```python
from build123d import *

# Parameters (mm, degrees)
EXTRUDE_1_DEPTH     = 20
EXTRUDE_2_DEPTH     = 8
CUT_EXTRUDE_1_DEPTH = 35.756294394
SKETCH_4_R          = 1.6
CUT_EXTRUDE_2_DEPTH = 37.307712679


with BuildPart() as part:
    # ｽｹｯﾁ1 → ﾎﾞｽ - 押し出し1 (new body)
    with BuildSketch(Plane(origin=(0, 0, 0), x_dir=(1, 0, 0), z_dir=(0, 1, 0))):
        with BuildLine():
            Line((-4.5, -8.93028555), (-4.5, -18))
            Line((-4.5, -18), (4.5, -18))
            Line((4.5, -18), (4.5, -8.93028555))
            ThreePointArc((4.5, -8.93028555), (0, 10), (-4.5, -8.93028555))
        make_face()
    extrude(amount=EXTRUDE_1_DEPTH)

    # ｽｹｯﾁ2 → ﾎﾞｽ - 押し出し2 (add)
    with BuildSketch(Plane(origin=(0, 20, 0), x_dir=(1, 0, 0), z_dir=(0, 1, 0))):
        Polygon((0, 5.773502692), (-5, 2.886751346), (-5, -2.886751346), (0, -5.773502692), (5, -2.886751346), (5, 2.886751346), align=None)
    extrude(amount=EXTRUDE_2_DEPTH)

    # ｽｹｯﾁ3 → ｶｯﾄ - 押し出し1 (cut, through all)
    with BuildSketch(Plane(origin=(0, 28, 0), x_dir=(1, 0, 0), z_dir=(0, 1, 0))):
        with BuildLine():
            Line((-3.638778503, -18), (-0.312080176, -1.543771668))
            ThreePointArc((-0.312080176, -1.543771668), (0, 1.575), (0.312080176, -1.543771668))
            Line((0.312080176, -1.543771668), (3.638778503, -18))
            ThreePointArc((3.638778503, -18), (0, -18.364114708), (-3.638778503, -18))
        make_face()
    extrude(amount=-CUT_EXTRUDE_1_DEPTH, mode=Mode.SUBTRACT)

    # ｽｹｯﾁ4 → ｶｯﾄ - 押し出し2 (cut, through all)
    with BuildSketch(Plane.ZY.offset(4.5)):
        with Locations((13.465142775, 15)):
            Circle(SKETCH_4_R)
        with Locations((13.465142775, 5)):
            Circle(SKETCH_4_R)
    extrude(amount=-CUT_EXTRUDE_2_DEPTH, mode=Mode.SUBTRACT)


solid = part.part
```
Input: part model. Units: mm. Frame: model coordinates. A direction names the side the tool comes from. Give positions to 0.01 mm unless a question says otherwise; leave off trailing zeros. Order: outer loops, then holes, each group sorted by start corner. A loop starts at its lowest first (then second) coordinate and runs counter-clockwise, first axis right, second up. Notation, with made-up numbers: (45.5, 52) - (67.5, 52) arc R12 ccw to (67.5, 58) - close; hole circle Ø1 at (20, 22). An arc over 180 degrees is marked (long way). Use a Markdown table: item, result.
(1) Section query D-D (z = 10.5). Output: boundary loops of the cut face in (x, y), then the cut area to 3 significant figures.
Computed values:
| item | result |
|---|---|
| outline | (-4.5, 0) - (-2.12, 0) - (-2.12, 20) - (-4.5, 20) - close; (2.12, 0) - (4.5, 0) - (4.5, 20) - (2.12, 20) - close |
| area | 95.1 mm2 |
(2) Section query A-A (z = 0). Output: boundary loops of the cut face in (x, y) (3 decimals), then the cut area to 3 significant figures.
Computed values:
| item | result |
|---|---|
| outline | (-10, 0) - (-1.575, 0) - (-1.575, 28) - (-5, 28) - (-5, 20) - (-10, 20) - close; (1.575, 0) - (10, 0) - (10, 20) - (5, 20) - (5, 28) - (1.575, 28) - close |
| area | 392 mm2 |
(3) Pin query (flat end, axial travel): pin 1 (4.5 mm diameter, centred on y = 14, z = 12, fed in from +X); pin 2 (12 mm diameter, centred on x = 0.5, z = -0.5, fed in from -Y); pin 3 (5 mm diameter, centred on y = 15, z = 13.47, fed in from -X); pin 4 (4.5 mm diameter, centred on y = 25, z = 1.5, fed in from -X). Return the tip coordinate at first contact, or that it passes through.
Computed values:
| item | result |
|---|---|
| pin 1 | stops at x = 4.5 |
| pin 2 | stops at y = 0 |
| pin 3 | stops at x = -4.5 |
| pin 4 | stops at x = -5 |
(4) Draft query along Y for faces 5 (the flat face through (4, 20, 4)), 6 (the cylindrical face through (3.656, 15.07, 11.867)), 7 (the cylindrical face through (-3.686, 15.07, 11.867)), 8 (the flat face through (4.5, 10, 14)). Return one class per face: released by +Y, released by -Y, zero draft, split by the parting line, or undercut.
Computed values:
| item | result |
|---|---|
| face 5 | released by +Y |
| face 6 | undercut |
| face 7 | undercut |
| face 8 | zero draft |
(5) Access query for faces 1 (the flat face through (-4.5, 10, 13)), 2 (the flat face through (-3.05, 23.944, 4.012)), 3 (the flat face through (2.535, 23.944, -4.31)), 4 (the flat face through (-2.465, 23.944, -4.35)). Directions: +Z, -Z, +X, -X, +Y, -Y. A direction counts if a zero-diameter tool reaches every point of the face in a straight line with its end or side. Return the directions, or none.
Computed values:
| item | result |
|---|---|
| face 1 | +Z, -X, +Y, -Y |
| face 2 | +Z, -X, +Y |
| face 3 | -Z, +X, +Y |
| face 4 | -Z, -X, +Y |
(6) Section query B-B (y = 15). Output: boundary loops of the cut face in (x, z) (3 decimals).
Computed values:
| item | result |
|---|---|
| outline | (-4.5, 8.93) arc R10 ccw (long way) to (4.5, 8.93) - (4.5, 11.865) - (2.399, 11.865) - (0.312, 1.544) arc R1.575 cw (long way) to (-0.312, 1.544) - (-2.399, 11.865) - (-4.5, 11.865) - close; (-4.5, 15.065) - (-3.045, 15.065) - (-3.639, 18) - (-4.5, 18) - close; (3.045, 15.065) - (4.5, 15.065) - (4.5, 18) - (3.639, 18) - close |
(7) Section query C-C (y = 3). Output: boundary loops of the cut face in (x, z) (3 decimals).
Computed values:
| item | result |
|---|---|
| outline | (-4.5, 8.93) arc R10 ccw (long way) to (4.5, 8.93) - (4.5, 18) - (3.639, 18) - (0.312, 1.544) arc R1.575 cw (long way) to (-0.312, 1.544) - (-3.639, 18) - (-4.5, 18) - close |
(8) Line query: line 1 (X direction, y = 14, z = 0) (3 decimals); line 2 (Y direction, x = -5.25, z = 6); line 3 (X direction, y = 3, z = 11). Output: solid intervals per line, ascending. Write a range as from..to.
Computed values:
| item | result |
|---|---|
| line 1 | x = -10..-1.575, 1.575..10 |
| line 2 | y = 0..20 |
| line 3 | x = -4.5..-2.22, 2.22..4.5 |
